```python
from build123d import *

# Parameters (mm, degrees)
F0_R     = 22.4155
F1_DEPTH = 7.62
F2_R     = 12.065
F3_DEPTH = 25.4
F5_DEPTH = 20.32
F6_R     = 5.08
F7_R     = 1.27
F8_R     = 1.4605
F9_DEPTH = 76.2
F11_SIZE = 1.27


# Not quite as in the source:
# - a fillet or chamfer that OpenCascade refuses, or shapes differently, is made with other operations: its cross-section is extruded or revolved along the edge and cut away or added


with BuildPart() as f1:
    # F0 (on Top) → F1 (new body)
    with BuildSketch(Plane.XY):
        with Locations((-27.5733582675, -25.1242369413)):
            Circle(F0_R)
    extrude(amount=F1_DEPTH)

    # F2 (on face) → F3 (cut)
    with BuildSketch(Plane.XY.offset(7.62)):
        with BuildLine():
            add(Edge.make_bspline(
                [(-22.4933582675, -7.3442369413), (-22.4933582675, -2.7248574376), (-30.1133582675, -5.0345471894), (-37.7333582675, -7.3442369413), (-30.1133582675, -9.6539266932), (-22.4933582675, -11.9636164451), (-22.4933582675, -7.3442369413)],
                knots=[0, 0, 0, 2.0943951024, 2.0943951024, 4.1887902048, 4.1887902048, 6.2831853072, 6.2831853072, 6.2831853072], degree=2, weights=[1, 0.5, 1, 0.5, 1, 0.5, 1]))
        make_face()
        with Locations((-27.5733582675, -25.1242369413)):
            Circle(F2_R)
    extrude(amount=-F3_DEPTH, mode=Mode.SUBTRACT)

    # F4 (on face) → F5 (join)
    with BuildSketch(Plane.XY.offset(7.62)):
        Polygon((-39.6383582675, -34.6492369413), (-39.6383582675, -25.1242369413), (-39.6383582675, -15.5992369413), (-47.2583582675, -15.5992369413), (-47.2583582675, -34.6492369413), align=None)
        Polygon((-7.8883582675, -34.6492369413), (-7.8883582675, -15.5992369413), (-15.5083582675, -15.5992369413), (-15.5083582675, -25.1242369413), (-15.5083582675, -34.6492369413), align=None)
    extrude(amount=F5_DEPTH)

    # F6
    f6_edges = [f1.edges().sort_by_distance(p)[0] for p in [
        (-11.698358, -34.649237, 27.94),
        (-11.698358, -15.599237, 27.94),
        (-43.448358, -34.649237, 27.94),
        (-43.448358, -15.599237, 27.94),
    ]]
    fillet(f6_edges, radius=F6_R)

    # F7
    f7_edges = [f1.edges().sort_by_distance(p)[0] for p in [
        (-7.888358, -34.649237, 15.24),
        (-47.258358, -15.599237, 15.24),
        (-47.258358, -34.649237, 15.24),
        (-47.258358, -33.161339, 26.452102),
        (-47.258358, -25.124237, 27.94),
        (-47.258358, -17.087134, 26.452102),
        (-7.888358, -33.161339, 26.452102),
        (-7.888358, -25.124237, 27.94),
        (-7.888358, -15.599237, 15.24),
        (-7.888358, -17.087134, 26.452102),
    ]]
    fillet(f7_edges, radius=F7_R)

    # F8 (on face) → F9 (cut)
    with BuildSketch(Plane(origin=(-47.2583582675, 0, 0), x_dir=(0, -1, 0), z_dir=(-1, 0, 0))):
        with Locations((20.8697369413, 19.05)):
            Circle(F8_R)
        with Locations((29.3787369413, 19.05)):
            Circle(F8_R)
    extrude(amount=-F9_DEPTH, mode=Mode.SUBTRACT)

    # F10: fillet of radius 2.54 on 1 edges, made by hand

    # F10_s1 → F10_t2 (revolve, cut)
    with BuildSketch(Plane.XZ.offset(25.1242369413)):
        with BuildLine():
            ThreePointArc((-5.1578582675, 2.54), (-5.9018070433, 0.7439487758), (-7.6978582675, 0))
            Line((-7.6978582675, 0), (-7.6978582675, -0.0508))
            Line((-7.6978582675, -0.0508), (-5.1070582675, -0.0508))
            Line((-5.1070582675, -0.0508), (-5.1070582675, 2.54))
            Line((-5.1070582675, 2.54), (-5.1578582675, 2.54))
        make_face()
    revolve(axis=Axis((-27.5733582675, -25.1242369413, 0), (0, 0, 1)), mode=Mode.SUBTRACT)

    # F11
    f11_edges = [f1.edges().sort_by_distance(p)[0] for p in [
        (-39.638358, -25.124237, 0),
    ]]
    chamfer(f11_edges, length=F11_SIZE)


solid = f1.part
```
The model under review builds one solid part; all positions refer to its coordinate system, in mm. A direction names the side the tool comes from. Give positions to 0.01 mm unless a question says otherwise; leave off trailing zeros. Write each loop counter-clockwise with the first axis right and the second up, starting at its lowest first coordinate (ties: lowest second). Pieces come first, ordered by that corner, then holes.
(1) For P1, Ø15, axis at y = -22.5, z = 18.5, coming from the +X side; P2, Ø15, axis at y = -25.5, z = 20.5, coming from the -X side; P3, Ø3, axis at x = -11.5, z = 19, coming from the +Y side; P4, Ø2.5, axis at y = -29.38, z = 19.05, coming from the +X side, all flat-tipped, find the tip position at first contact; note any pin that passes through.
(2) Consider section A-A, the plane z = 19.05. Give the boundary of the cut face in (x, y), and give its area (3 significant figures).
(3) Consider section B-B, the plane z = 9.25. Give the boundary of the cut face in (x, y).
(4) To check wall thickness, follow L1, parallel to X at y = -22, z = 26.75; L2, parallel to X at y = -33.5, z = 23.5; L3, parallel to Y at x = -41.5, z = 19.5. State the ranges of each line that lie inside material, in increasing order.
(5) Consider section C-C, the plane x = -43. Give the number of separate pieces and of enclosed holes in the cut face, and give its area (3 significant figures).
(6) The part is to be moulded in two halves that separate along Y. For faces 6 (the cylindrical face through (-42.858, -17.048, 26.412)), 7 (the cylindrical face through (-46.876, -34.287, 15.133)), 8 (the flat face through (-23, -38, 0)), 9 (the cylindrical face through (-43.502, -30.053, 17.754)), say which applies: released by +Y, released by -Y, zero draft, split by the parting line, or undercut.
(7) Tool access review of faces 1 (the cylindrical face through (-8.27, -34.287, 15.347)), 2 (the flat face through (-47.258, -25, 17)), 3 (the flat face through (-12, -15.599, 15)), 4 (the cylindrical face through (-8.27, -15.96, 15.13)), 5 (the flat face through (-12, -34.649, 15)): name each direction out of +Z, -Z, +X, -X, +Y, -Y from which nothing blocks a thin tool from reaching the whole face with its end or side.
Returned:
1. P1: stops at x = -7.89
1. P2: stops at x = -47.26
1. P3: stops at y = -15.6
1. P4: passes through
2. outline: (-47.26, -33.38) arc R1.27 ccw to (-45.99, -34.65) - (-39.64, -34.65) - (-39.64, -30.84) - (-47.26, -30.84) - close; (-47.26, -27.92) - (-39.64, -27.92) - (-39.64, -22.33) - (-47.26, -22.33) - close; (-47.26, -19.41) - (-39.64, -19.41) - (-39.64, -15.6) - (-45.99, -15.6) arc R1.27 ccw to (-47.26, -16.87) - close; (-15.51, -34.65) - (-9.16, -34.65) arc R1.27 ccw to (-7.89, -33.38) - (-7.89, -30.84) - (-15.51, -30.84) - close; (-15.51, -27.92) - (-7.89, -27.92) - (-7.89, -22.33) - (-15.51, -22.33) - close; (-15.51, -19.41) - (-7.89, -19.41) - (-7.89, -16.87) arc R1.27 ccw to (-9.16, -15.6) - (-15.51, -15.6) - close
2. area: 200 mm2
3. outline: (-47.26, -33.38) arc R1.27 ccw to (-45.99, -34.65) - (-39.64, -34.65) - (-39.64, -15.6) - (-45.99, -15.6) arc R1.27 ccw to (-47.26, -16.87) - close; (-15.51, -34.65) - (-9.16, -34.65) arc R1.27 ccw to (-7.89, -33.38) - (-7.89, -16.87) arc R1.27 ccw to (-9.16, -15.6) - (-15.51, -15.6) - close
4. L1: x = -47.26 to -39.64, -15.51 to -7.89
4. L2: x = -47.25 to -39.64, -15.51 to -7.9
4. L3: y = -34.65 to -30.77, -27.99 to -22.26, -19.48 to -15.6
5. separate pieces: 1
5. enclosed holes: 2
5. area: 607 mm2
6. face 6: released by +Y
6. face 7: released by -Y
6. face 8: zero draft
6. face 9: undercut
7. face 1: +Z, +X, -Y
7. face 2: +Z, -X, +Y, -Y
7. face 3: +Z, +X, -X, +Y
7. face 4: +Z, +X, +Y
7. face 5: +Z, +X, -X, -Y
